Build history of the part. All positions in model axes, mm. Face numbers are marked on the shaded views. A direction names the side the tool comes from. Round coordinates to 2 decimals unless told otherwise and drop trailing zeros. Write each loop counter-clockwise with the first axis right and the second up, starting at its lowest first coordinate (ties: lowest second). Pieces come first, ordered by that corner, then holes.
1) Saw through at A-A (z = 2.45). Write the cut outline in (x, y).
2) Saw through at C-C (x = 0.3). Write the cut outline in (y, z).
3) Saw through at B-B (y = -16.5). Write the cut outline in (x, z).
4) Pull direction X, two halves, no side cores. Call the marked faces 1, 2 and 3: +X half, -X half, draft (parallel to the pull), parting line (faces both ways), or undercut.
5) Which spindle directions (+Z, -Z, +X, -X, +Y, -Y) get a long thin tool onto all of the face, cutting with end or side? Do the marked faces 4 and 5. Say none if no direction does.
6) Flat gauge pin, fed straight in: pin 1 (1 mm diameter, centred on x = 0, y = -7.5, fed in from +Z). Where does the tip first touch, or does it go through?
7) Wall check: probe 1 along X at (y, z) = (-1.75, 1.65); probe 2 along X at (y, z) = (-9, 2.05); probe 3 along Z at (x, y) = (1.8, -7.5). Give the ranges that are in metal, low to high.
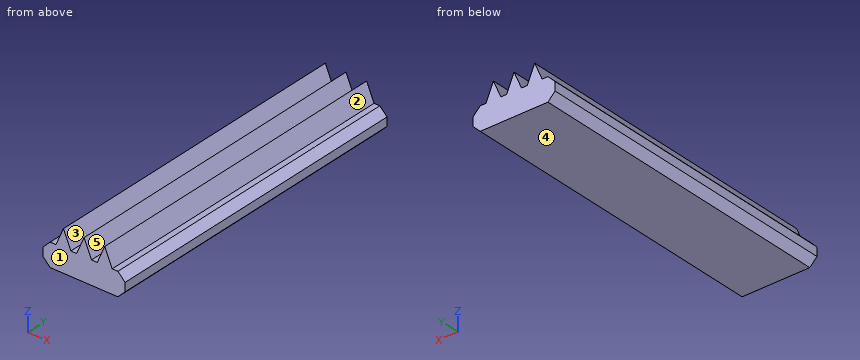
from build123d import *

# Parameters (mm, degrees)
SKETCH014_W     = 5.7
SKETCH014_H     = 1.6
PAD004_DEPTH    = 22
PAD005_DEPTH    = 22
CHAMFER002_SIZE = 0.5


with BuildPart() as part:
    # Sketch014 → Pad004 (new body)
    with BuildSketch(Plane.XZ):
        with Locations((0, 0.8)):
            Rectangle(SKETCH014_W, SKETCH014_H)
    extrude(amount=PAD004_DEPTH)

    # Sketch015 → Pad005 (join)
    with BuildSketch(Plane.XZ):
        Polygon((0.516667, 1.6), (0, 2.8), (-0.516667, 1.6), align=None)
        Polygon((-0.916667, 1.6), (-1.433333, 2.8), (-1.95, 1.6), align=None)
        Polygon((0.916667, 1.6), (1.433333, 2.8), (1.95, 1.6), align=None)
    extrude(amount=PAD005_DEPTH)

    # Chamfer002
    chamfer002_edges = [part.edges().sort_by_distance(p)[0] for p in [
        (-2.85, -11, 1.6),
        (-2.85, -11, 0),
        (2.85, -11, 0),
        (2.85, -11, 1.6),
    ]]
    chamfer(chamfer002_edges, length=CHAMFER002_SIZE)


solid = part.part
Evaluation:
1. outline: (-1.58, -22) - (-1.28, -22) - (-1.28, 0) - (-1.58, 0) - close; (-0.15, -22) - (0.15, -22) - (0.15, 0) - (-0.15, 0) - close; (1.28, -22) - (1.58, -22) - (1.58, 0) - (1.28, 0) - close
2. outline: (-22, 0) - (0, 0) - (0, 2.1) - (-22, 2.1) - close
3. outline: (-2.85, 0.5) - (-2.35, 0) - (2.35, 0) - (2.85, 0.5) - (2.85, 1.1) - (2.35, 1.6) - (1.95, 1.6) - (1.43, 2.8) - (0.92, 1.6) - (0.52, 1.6) - (0, 2.8) - (-0.52, 1.6) - (-0.92, 1.6) - (-1.43, 2.8) - (-1.95, 1.6) - (-2.35, 1.6) - (-2.85, 1.1) - close
4. face 1: draft
4. face 2: +X half
4. face 3: undercut
5. face 4: -Z, +X, -X, +Y, -Y
5. face 5: +Z, +Y, -Y
6. pin 1: stops at z = 2.8
7. probe 1: x = -1.93 to -0.94, -0.5 to 0.5, 0.94 to 1.93
7. probe 2: x = -1.76 to -1.11, -0.32 to 0.32, 1.11 to 1.76
7. probe 3: z = 0 to 1.95
